from build123d import *

# Parameters (mm, degrees)
BOSS_EXTRUDE1_DEPTH = 2
SKETCH2_W           = 20
SKETCH2_H           = 65
CUT_EXTRUDE1_DEPTH  = 115.109502301


with BuildPart() as part:
    # Sketch1 → Boss-Extrude1 (new body)
    with BuildSketch(Plane(origin=(0, 0, 0), x_dir=(0, 0, -1), z_dir=(1, 0, 0))):
        Polygon((-23.487008112, -53.123171146), (-23.487008112, 53.119179438), (-79.3154252, 49.479562724), (-80.828417088, 68.421259669), (80.828417088, 78.960138367), (82.341408976, 60.018441422), (26.512991888, 56.378824708), (26.512991888, -56.378824708), (81.84341634, -59.981558578), (81.107293536, -78.973862025), (-80.550377935, -68.447834544), (-78.817432564, -49.520437276), align=None)
    extrude(amount=BOSS_EXTRUDE1_DEPTH)

    # Sketch2 → Cut-Extrude1 (cut, through all)
    with BuildSketch(Plane(origin=(2, 0, 0), x_dir=(0, 0, -1), z_dir=(1, 0, 0))):
        with Locations((1.46172303, 23.500819189)):
            Rectangle(SKETCH2_W, SKETCH2_H)
    extrude(amount=-CUT_EXTRUDE1_DEPTH, mode=Mode.SUBTRACT)


solid = part.part
Can you work these out from the model? Positions are in its coordinate system, mm. A direction names the side the tool comes from. Give positions to 0.01 mm unless a question says otherwise; leave off trailing zeros. Loops run counter-clockwise (first coordinate to the right, second up) from the corner with the lowest first, then second, coordinate; pieces in that order, holes last. Notation, with made-up numbers: (-40, 31.25) -> (12, 31.25) arc R20 cw to (12, 53.25) -> close; hole circle Ø7 at (79.25, 20). An arc over 180 degrees is marked (long way). Use one line per item in the form item = value.
1) If we section it at A-A (y = 13): Please give me the cut outline in (x, z).
Answers:
outline = (0, -26.51) -> (2, -26.51) -> (2, -11.46) -> (0, -11.46) -> close; (0, 8.54) -> (2, 8.54) -> (2, 23.49) -> (0, 23.49) -> close
2) I need wall thicknesses on line 1 along Z through (x, y) = (1.7, 35); line 2 along Y through (x, z) = (1.6, -65); line 3 along Z through (x, y) = (0.6, -32.5). Which ranges of each line are inside material? Lowest first, please.
Answers:
line_1 = -26.51 to -11.46, 8.54 to 23.49
line_2 = -77.93 to -58.88, 58.89 to 77.93
line_3 = -26.51 to 23.49
3) For faces 4 (the face through (0.986, -58.155, -53.791)), 5 (the face through (0.986, 73.617, 1.132)), 6 (the face through (0.986, 51.325, 51.01)), which set-ups out of +Z, -Z, +X, -X, +Y, -Y let a thin tool reach every point of the face, with its end or its side?
Answers:
face_4 = -Z, +X, -X
face_5 = +Z, +X, -X, +Y
face_6 = +X, -X
4) We'd pull the mould along Z, two halves only. Please class faces 1 (the face through (2, -16, -2)), 2 (the face through (0.986, 58.224, -54.818)), 3 (the face through (1, -51.3, 51.5)): released by +Z, released by -Z, zero draft, split by the parting line, or undercut.
Answers:
face_1 = zero draft
face_2 = released by -Z
face_3 = undercut
5) If we section it at B-B (x = 1.3): Please give me the cut outline in (y, z), plus the area to 3 significant figures.
Answers:
outline = (-78.97, -81.11) -> (-59.98, -81.84) -> (-56.38, -26.51) -> (56.38, -26.51) -> (60.02, -82.34) -> (78.96, -80.83) -> (68.42, 80.83) -> (49.48, 79.32) -> (53.12, 23.49) -> (-53.12, 23.49) -> (-49.52, 78.82) -> (-68.45, 80.55) -> close; hole (-9, -11.46) -> (56, -11.46) -> (56, 8.54) -> (-9, 8.54) -> close
area = 10,300 mm²
6) If we section it at C-C (z = -5): Please give me the cut outline in (x, y), plus the area to 3 significant figures.
Answers:
outline = (0, -74.02) -> (2, -74.02) -> (2, -9) -> (0, -9) -> close; (0, 56) -> (2, 56) -> (2, 74.02) -> (0, 74.02) -> close
area = 166 mm²
7) Will these pins go through, and if not, where does the flat tip stop? pin 1 (0.6 mm diameter, centred on x = 1, z = 1, fed in from +Y); pin 2 (1 mm diameter, centred on x = 1.5, y = -54.5, fed in from +Z); pin 3 (0.6 mm diameter, centred on x = 1, y = 29, fed in from +Z).
Answers:
pin_1 = 73.65
pin_2 = 79.32
pin_3 = 23.49
8) If we section it at D-D (z = 18.5): Please give me the cut outline in (x, y), plus the area to 3 significant figures.
Answers:
outline = (0, -72.49) -> (2, -72.49) -> (2, 72.48) -> (0, 72.48) -> close
area = 290 mm²
